CAD build for the part. Positions are in the model's coordinates, mm. Face numbers are marked on the shaded views. A direction names the side the tool comes from. Round coordinates to 2 decimals unless told otherwise and drop trailing zeros. Order: outer loops, then holes, each group sorted by start corner. A loop starts at its lowest first (then second) coordinate and runs counter-clockwise, first axis right, second up. Notation, with made-up numbers: M 18,65 L 65,65 A20 cw 65,81 Z; hole C 70,-25.75 d5. An arc over 180 degrees is marked long. Put each result on its own line as item: value.
Autodesk Inventor part; units mm, degrees
ref_plane "YZ Plane" through (0, 0, 0) normal (1, 0, 0) x (0, 1, 0)
ref_plane "XZ Plane" through (0, 0, 0) normal (0, 1, 0) x (-1, 0, 0)
ref_plane "XY Plane" through (0, 0, 0) normal (0, 0, 1) x (1, 0, 0)
sketch "Szkic1" plane through (0, 0, 0) normal (0, 0, 1) x (1, 0, 0)
  circle A0 centre (26.2, 0.975) radius 1.45
  circle A1 centre (26.2, 0.975) radius 3
  line L0 (29.2, 0.975) -> (29.2, -8.7925)
  line L1 (23.2, -14.7925) -> (20.5681, -14.7925)
  line L2 (17.1107, -9.0757) -> (21.2, -9.0757)
  line L3 (23.2, -7.0757) -> (23.2, 0.975)
  line L4 (18.2447, -12.1144) -> (21.525, -14.6291)
  line L5 (16.8275, -11.925) -> (-16.8275, 13.875) construction
  line L6 (20.0699, -9.7335) -> (23.3502, -12.2482)
  line L7 (18.2447, -12.1144) -> (20.0699, -9.7335)
  line L8 (21.525, -14.6291) -> (23.3502, -12.2482)
  line L9 (29.2, -8.7925) -> (23.2, -14.7925)
  line L10 (15.6301, -11.0071) -> (17.1107, -9.0757)
  line L11 (21.2, -9.0757) -> (23.2, -7.0757)
  line L12 (15.6301, -11.0071) -> (20.5681, -14.7925)
  point P0 (0, 0)
  point P1 (29.2, -14.7925)
  point P2 (18.5681, -14.7925)
  point P3 (15.1107, -9.0757)
  point P4 (23.2, -9.0757)
  point P5 (18.9313, -9.4578)
  point P6 (19.7101, -9.4578)
  dimension "d0" = 3
  dimension "d5" = 6
  dimension "d6" = 6
  dimension "d7" = 2
  dimension "d9" = 2
  dimension "d10" = 2
  dimension "d11" = 2
  dimension "d12" = 2
  dimension "d13" = 6
extrude "Wyciągnięcie proste1" add sketch "Szkic1" along normal blind 4 contours A1 | L0 L9 L1 L12 L10 L2 L11 L3 A1 | L7 L6 L8 L4
sketch "Szkic4" plane through (0, 0, 4) normal (0, 0, 1) x (1, 0, 0)
  line L0 (22.5711, -12.1912) -> (17.6276, -8.4015)
  line L1 (16.8275, -11.925) -> (-16.8275, 13.875) construction
  line L2 (17.6276, -8.4015) -> (15.6301, -11.0071)
  line L3 (15.6301, -11.0071) -> (20.5737, -14.7968)
  line L4 (20.5737, -14.7968) -> (22.5711, -12.1912)
  line L5 (15.6301, -11.0071) -> (20.5681, -14.7925)
  line L6 (17.1107, -9.0757) -> (15.6301, -11.0071)
  point P0 (0, 0)
extrude "Wyciągnięcie proste2" add sketch "Szkic4" along normal blind 4 and the other way blind 4
sketch "Szkic5" plane through (20.5737, -14.7968, 0) normal (-0.6084, -0.7936, 0) x (0.7936, -0.6084, 0)
  circle A0 centre (-3.229, 5) radius 1.45
  line L0 (-6.229, 0) -> (-6.229, 8)
  line L1 (-6.229, 8) -> (0, 8)
  point P0 (-25.3303, 0)
  dimension "d16" = 3
  dimension "d17" = 3
  dimension "d18" = 2.9
extrude "Wyciągnięcie proste3" cut sketch "Szkic5" against normal blind 4.25
properties part number "mirror_arm"
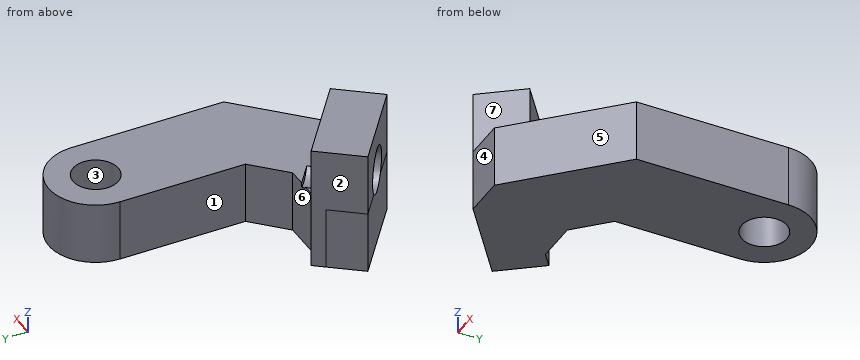
Item 1: Band-saw the part on A-A on x = 26.2. Give the cut face in (y, z) (1 decimal).
Answers below:
outline: M -11.8,0 L -0.5,0 L -0.5,4 L -11.8,4 Z; M 2.4,0 L 4,0 L 4,4 L 2.4,4 Z
Item 2: Tool access for the marked faces 5, 6 and 7: list every direction of +Z, -Z, +X, -X, +Y, -Y with a clear straight run to the whole face (end or side of a thin tool).
Answers below:
face 5: +Z, -Z, +X, -Y
face 6: +Z, -Z, +Y
face 7: +Z, +X, -Y
Item 3: Pin check, flat tips, straight feed: P1, Ø2, axis at x = 20, z = 2.5, coming from the +Y side; P2, Ø4.5, axis at y = -2.5, z = 2.5, coming from the -X side; P3, Ø0.8, axis at x = 21.5, z = 2, coming from the -Y side. Stop position of each tip, or through.
Answers below:
P1: y = -9.08
P2: x = 23.2
P3: y = -14.79
Item 4: Probe line 1 along X through (y, z) = (-2.25, 2.25); line 2 along Y through (x, z) = (26.25, 3.75); line 3 along Z through (x, y) = (25.25, -4.75). List the from-to ranges inside material, lowest first. Write a range as [from, to].
Answers below:
line 1: [23.2, 29.2]
line 2: [-11.74, -0.47], [2.42, 3.97]
line 3: [0, 4]
Item 5: Band-saw the part on D-D on y = -1.25. Give the cut face in (x, z).
Answers below:
outline: M 23.2,0 L 29.2,0 L 29.2,4 L 23.2,4 Z
Item 6: Band-saw the part on C-C on z = 5.5. Give the cut face in (x, y).
Answers below:
outline: M 15.63,-11.01 L 16.93,-12 L 18.93,-9.4 L 17.63,-8.4 Z; M 19.09,-13.66 L 20.57,-14.8 L 22.57,-12.19 L 21.09,-11.05 Z
Item 7: Mould opens along Y. For the marked faces 1, 2, 3 and 4 say: pulls with the +Y half, pulls with the -Y half, needs draft (parallel to the pull), parting line crosses it, or undercut.
Answers below:
face 1: needs draft
face 2: pulls with the +Y half
face 3: undercut
face 4: pulls with the -Y half
